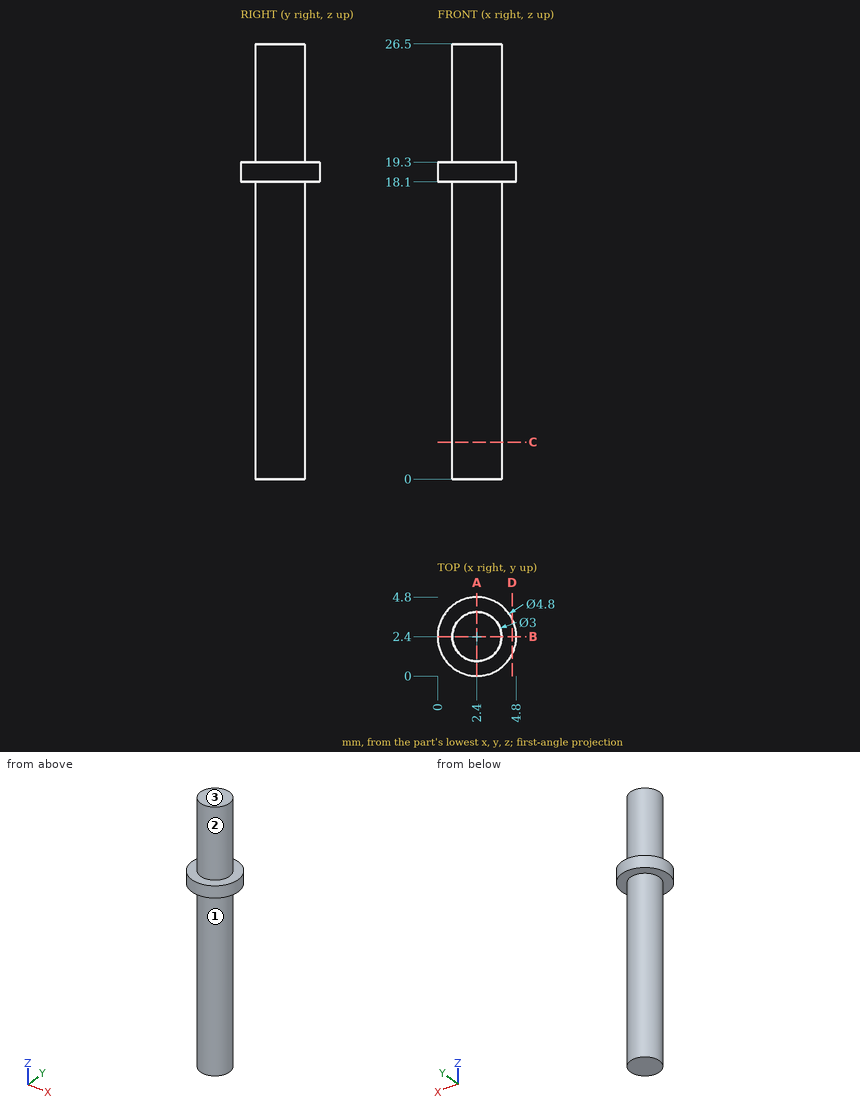
Print and shaded views of the part. All mm, measured from the part's lowest x, y and z. A direction names the side the tool comes from. Round coordinates to 2 decimals unless told otherwise and drop trailing zeros. Loops run counter-clockwise (first coordinate to the right, second up) from the corner with the lowest first, then second, coordinate; pieces in that order, holes last. Notation, with made-up numbers: (23.25, 87.25) -> (72.25, 87.25) arc R7 ccw to (72.25, 95.25) -> close; hole circle Ø9 at (-32, 25.5). An arc over 180 degrees is marked (long way). Use CSV: the item, a comma, the result in double quotes. Start each with the question number.
1) Wall check: L1, parallel to Z at x = 1.5, y = 0.85; L2, parallel to X at y = 3.25, z = 21.25; L3, parallel to Y at x = 3.45, z = 21. Give the ranges that are in metal, low to high. Write a range as [from, to].
2) Which spindle directions (+Z, -Z, +X, -X, +Y, -Y) get a long thin tool onto all of the face, cutting with end or side? Do the marked faces 1, 2 and 3. Say none if no direction does.
3) Cut at D-D, the plane x = 4.55. Write the cut outline in (y, z).
4) Cut at C-C, the plane z = 2.25. Write the cut outline in (x, y), plus the area to 3 significant figures.
5) Drop flat-ended pins along their axis: P1, Ø1.5, axis at y = 2.5, z = 5, coming from the +X side; P2, Ø1.5, axis at y = 1.5, z = 6.5, coming from the -X side. Give the stop position or say it passes through.
6) Cut at A-A, the plane x = 2.4. Write the cut outline in (y, z).
Determined:
1,L1,"z = [18.1, 19.3]"
1,L2,"x = [1.16, 3.64]"
1,L3,"y = [1.33, 3.47]"
2,face 1,"-Z"
2,face 2,"+Z"
2,face 3,"+Z, +X, -X, +Y, -Y"
3,outline,"(1.33, 18.1) -> (3.47, 18.1) -> (3.47, 19.3) -> (1.33, 19.3) -> close"
4,outline,"circle Ø3 at (2.4, 2.4)"
4,area,"7.07 mm2"
5,P1,"stops at x = 3.9"
5,P2,"stops at x = 0.91"
6,outline,"(0, 18.1) -> (0.9, 18.1) -> (0.9, 0) -> (3.9, 0) -> (3.9, 18.1) -> (4.8, 18.1) -> (4.8, 19.3) -> (3.9, 19.3) -> (3.9, 26.5) -> (0.9, 26.5) -> (0.9, 19.3) -> (0, 19.3) -> close"
